Read the model definition and answer for the solid it produces. Units are mm, in the model's axes. Face numbers are marked on the shaded views. A direction names the side the tool comes from. Give positions to 0.01 mm unless a question says otherwise; leave off trailing zeros. Loops run counter-clockwise (first coordinate to the right, second up) from the corner with the lowest first, then second, coordinate; pieces in that order, holes last. Notation, with made-up numbers: (31.25, -33) - (65.25, -33) arc R9 ccw to (65.25, -16) - close; hole circle Ø4 at (65.25, 68.25). An arc over 180 degrees is marked (long way). Write each question's results on one line, items separated by ' | '. Start each with the question number.
Q1. The part is cut by section A-A, the plane z = 15.5. Write down the section's boundary in (x, y) (3 decimals), plus the area to 3 significant figures.
Q2. Find the intervals of material crossed by line 1 (Y direction, x = -0.5, z = 6); line 2 (Y direction, x = 0, z = 14.5); line 3 (Z direction, x = -11.5, y = 2), in increasing order. Write a range as from..to.
Q3. The part is cut by section D-D, the plane z = 23.5. Write down the section's boundary in (x, y), plus the area to 3 significant figures.
Q4. Determine the mould class of the marked faces 3, 4 and 5 for opening direction X: +X half, -X half, draft (parallel to the pull), parting line (faces both ways), or undercut.
Q5. The part is cut by section C-C, the plane z = 7.25. Write down the section's boundary in (x, y) (3 decimals).
Q6. The part is cut by section B-B, the plane y = 0. Write down the section's boundary in (x, z), plus the area to 3 significant figures.
Q7. Given pin 1 (13 mm diameter, centred on x = -0.5, y = 4.5, fed in from -Z); pin 2 (1.1 mm diameter, centred on y = -17, z = 13, fed in from +X); pin 3 (6 mm diameter, centred on x = -2, z = 16.5, fed in from -Y), each flat-ended and moving along its own axis, determine where each tip first touches the part or whether it passes through.
Q8. For the marked faces 1 and 2, determine the directions among +Z, -Z, +X, -X, +Y, -Y from which every point of the face is accessible in a straight line to the end or side of a thin tool.
```python
from build123d import *

# Parameters (mm, degrees)
F3_W       = 0.75
F3_H       = 1.9961989338
F5_SIZE2   = 8.144336
F5_SIZE    = 0.99999
F5_2_SIZE2 = 8.144336
F5_2_SIZE  = 0.99999
F5_3_SIZE2 = 8.144336
F5_3_SIZE  = 0.99999


# Not quite as in the source:
# - a fillet or chamfer is up to 0.001 mm smaller than in the source, because OpenCascade refuses the exact size


with BuildPart() as f1:
    # F0 (on Front) → F1 (revolve)
    with BuildSketch(Plane.XZ):
        Polygon((16.5, 25), (0, 25), (0, 23), (12.8431457505, 23), (17.5, 18.3431457505), (17.5, 1), (18.5, 0), (19.5, 0), (19.5, 22), align=None)
    revolve(axis=Axis((0, 0, 16.9686058983), (0, 0, 1)))

    # F3 (on offset) → F4 (join, up to the next surface of F1)
    with BuildSketch(Plane.XY.offset(2)):
        with Locations((0, -17.4980994669)):
            Rectangle(F3_W, F3_H)
        Polygon((16.2056781502, 8.9233399405), (15.8306781502, 9.5728589933), (14.1019191624, 8.5747595264), (14.4769191624, 7.9252404736), align=None)
        Polygon((-15.8306781502, 9.5728589933), (-16.2056781502, 8.9233399405), (-14.4769191624, 7.9252404736), (-14.1019191624, 8.5747595264), align=None)
    extrude(until=Until.NEXT)

    # F5 (size 1 and 8.144346428 in the source; OpenCascade refuses exactly that, so slightly less here)
    f5_edges = [f1.edges().sort_by_distance(p)[0] for p in [
        (0, -16.5, 2),
    ]]
    f5_side = f1.faces().sort_by_distance((0, -16.999331, 2))[0]
    chamfer(f5_edges, length=F5_SIZE, length2=F5_SIZE2, reference=f5_side)

    # F5#2 (size 1 and 8.144346428 in the source; OpenCascade refuses exactly that, so slightly less here)
    f5_2_edges = [f1.edges().sort_by_distance(p)[0] for p in [
        (14.289419, 8.25, 2),
    ]]
    f5_2_side = f1.faces().sort_by_distance((14.721853, 8.499666, 2))[0]
    chamfer(f5_2_edges, length=F5_2_SIZE, length2=F5_2_SIZE2, reference=f5_2_side)

    # F5#3 (size 1 and 8.144346428 in the source; OpenCascade refuses exactly that, so slightly less here)
    f5_3_edges = [f1.edges().sort_by_distance(p)[0] for p in [
        (-14.289419, 8.25, 2),
    ]]
    f5_3_side = f1.faces().sort_by_distance((-14.721853, 8.499666, 2))[0]
    chamfer(f5_3_edges, length=F5_3_SIZE, length2=F5_3_SIZE2, reference=f5_3_side)


solid = f1.part
```
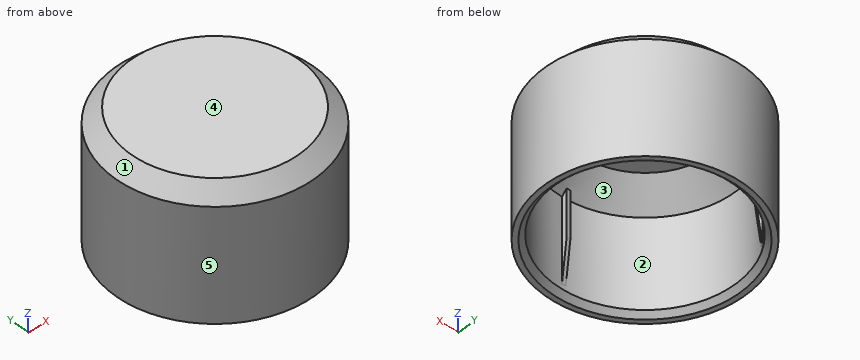
Check sheet entries:
1) outline: circle Ø39 at (0, 0); hole (-15.339, 8.423) arc R17.5 ccw to (-0.375, -17.496) - (-0.375, -16.5) - (0.375, -16.5) - (0.375, -17.496) arc R17.5 ccw to (15.339, 8.423) - (14.477, 7.925) - (14.102, 8.575) - (14.964, 9.073) arc R17.5 ccw to (-14.964, 9.073) - (-14.102, 8.575) - (-14.477, 7.925) - close | area: 235 mm^2
2) line 1: y = -19.49..-17.49, 17.49..19.49 | line 2: y = -19.5..-16.5, 17.5..19.5 | line 3: z = 23..25
3) outline: circle Ø36 at (0, 0) | area: 1,020 mm^2
4) face 3: undercut | face 4: draft | face 5: parting line
5) outline: circle Ø39 at (0, 0); hole (-15.339, 8.423) arc R17.5 ccw to (-0.375, -17.496) - (-0.375, -16.855) - (0.375, -16.855) - (0.375, -17.496) arc R17.5 ccw to (15.339, 8.423) - (14.785, 8.103) - (14.41, 8.752) - (14.964, 9.073) arc R17.5 ccw to (-14.964, 9.073) - (-14.41, 8.752) - (-14.785, 8.103) - close
6) outline: (-19.5, 0) - (-18.5, 0) - (-17.5, 1) - (-17.5, 18.34) - (-12.84, 23) - (12.84, 23) - (17.5, 18.34) - (17.5, 1) - (18.5, 0) - (19.5, 0) - (19.5, 22) - (16.5, 25) - (-16.5, 25) - (-19.5, 22) - close | area: 182 mm^2
7) pin 1: stops at z = 23 | pin 2: stops at x = 10.47 | pin 3: stops at y = -19.5
8) face 1: +Z | face 2: -Z
